from build123d import *

# Parameters (mm, degrees)
SKETCH_R     = 1.5
PAD_DEPTH    = 3
FILLET_R     = 4.99
FILLET001_R  = 3.49
PAD001_DEPTH = 5
CHAMFER_SIZE = 1.5


with BuildPart() as part:
    # Sketch → Pad (new body)
    with BuildSketch(Plane.XY):
        Polygon((-10.606602, 10.606602), (0, 0), (-10.606602, -10.606602), (-14.142136, -7.071068), (-24.571068, -17.5), (11, -17.5), (11, 17.5), (-24.571068, 17.5), (-14.142136, 7.071068), align=None)
        with Locations((5.5, 14)):
            Circle(SKETCH_R, mode=Mode.SUBTRACT)
        with Locations((5.5, -14)):
            Circle(SKETCH_R, mode=Mode.SUBTRACT)
    extrude(amount=PAD_DEPTH)

    # Fillet
    fillet_edges = [part.edges().sort_by_distance(p)[0] for p in [
        (-14.142136, -7.071068, 1.5),
        (-14.142136, 7.071068, 1.5),
    ]]
    fillet(fillet_edges, radius=FILLET_R)

    # Fillet001
    fillet001_edges = [part.edges().sort_by_distance(p)[0] for p in [
        (-24.571068, -17.5, 1.5),
        (-24.571068, 17.5, 1.5),
    ]]
    fillet(fillet001_edges, radius=FILLET001_R)

    # Sketch001 (on Face17 of Fillet001) → Pad001 (join)
    with BuildSketch(Plane.XY.offset(3)):
        Polygon((-9.5, 9.5), (11, 9.5), (11, -9.5), (-9.5, -9.5), (0, 0), align=None)
    extrude(amount=PAD001_DEPTH)

    # Chamfer
    chamfer_edges = [part.edges().sort_by_distance(p)[0] for p in [
        (4, -14, 3),
        (4, 14, 3),
    ]]
    chamfer(chamfer_edges, length=CHAMFER_SIZE)


solid = part.part
The listing builds one solid part. Answer for the finished solid, in the listing's coordinates (mm). A direction names the side the tool comes from. Coordinates: 2 decimals unless noted, no trailing zeros. Write each loop counter-clockwise with the first axis right and the second up, starting at its lowest first coordinate (ties: lowest second). Pieces come first, ordered by that corner, then holes. Notation, with made-up numbers: M -14,50.5 L 27,50.5 A8 cw 27,57.5 Z; hole C 1.5,-23.5 d3. An arc over 180 degrees is marked long. Use one line per item in the form item = value.
Item 1: Find section B-B, the plane y = 14. Give the vertices of the cut face in (x, z), plus the area to 3 significant figures.
Model answer:
outline = M -19.64,0 L 4,0 L 4,1.5 L 2.5,3 L -19.64,3 Z; M 7,0 L 11,0 L 11,3 L 8.5,3 L 7,1.5 Z
area = 80.7 mm2
Item 2: Find section C-C, the plane x = -13. Give the vertices of the cut face in (y, z), plus the area to 3 significant figures.
Model answer:
outline = M -17.5,0 L -9.27,0 L -9.27,3 L -17.5,3 Z; M 9.27,0 L 17.5,0 L 17.5,3 L 9.27,3 Z
area = 49.4 mm2
Item 3: Find section A-A, the plane x = 5.5. Give the vertices of the cut face in (y, z).
Model answer:
outline = M -17.5,0 L -15.5,0 L -15.5,1.5 L -17,3 L -17.5,3 Z; M -12.5,0 L 12.5,0 L 12.5,1.5 L 11,3 L 9.5,3 L 9.5,8 L -9.5,8 L -9.5,3 L -11,3 L -12.5,1.5 Z; M 15.5,0 L 17.5,0 L 17.5,3 L 17,3 L 15.5,1.5 Z
Item 4: Given P1, Ø2.5, axis at x = -9, y = 13.5, coming from the +Z side; P2, Ø2.5, axis at x = 1, z = 5.5, coming from the +Y side; P3, Ø3, axis at y = -7.5, z = 4.5, coming from the -X side, each flat-ended and moving along its own axis, determine where each tip first touches the part or whether it passes through.
Model answer:
P1 = 3
P2 = 9.5
P3 = -9
Item 5: For faces 1 (the face through (-14.09, 9.14, 1.52)), 2 (the face through (1, -9.5, 5)), 3 (the face through (1, 9.5, 5)), 4 (the face through (-18.15, 11.08, 1.48)), determine the directions among +Z, -Z, +X, -X, +Y, -Y from which every point of the face is accessible in a straight line to the end or side of a thin tool.
Model answer:
face_1 = +Z, -Z
face_2 = +Z, +X, -X, -Y
face_3 = +Z, +X, -X, +Y
face_4 = +Z, -Z, -X
Item 6: Find the intervals of material crossed by probe 1 along Y at (x, z) = (5.5, 1.1); probe 2 along Y at (x, z) = (6.5, 1.75); probe 3 along Z at (x, y) = (-6, -15), in increasing order.
Model answer:
probe_1 = -17.5 to -15.5, -12.5 to 12.5, 15.5 to 17.5
probe_2 = -17.5 to -15.44, -12.56 to 12.56, 15.44 to 17.5
probe_3 = 0 to 3
Item 7: Find section D-D, the plane z = 6.5. Give the vertices of the cut face in (x, y), plus the area to 3 significant figures.
Model answer:
outline = M -9.5,-9.5 L 11,-9.5 L 11,9.5 L -9.5,9.5 L 0,0 Z
area = 299 mm2
Item 8: The mould has two halves that part along X. Classify faces 5 (the face through (-3, -17.5, 1)), 6 (the face through (11, 0, 3)), 7 (the face through (4.3, -14.9, 0.7)), 8 (the face through (-14.09, -9.14, 1.52)): released by +X, released by -X, zero draft, split by the parting line, or undercut.
Model answer:
face_5 = zero draft
face_6 = released by +X
face_7 = undercut
face_8 = undercut
